Here's how the part is built. I have some questions about the finished solid (model axes, mm). Face numbers are marked on the shaded views. A direction names the side the tool comes from. Round coordinates to 2 decimals unless told otherwise and drop trailing zeros. Write each loop counter-clockwise with the first axis right and the second up, starting at its lowest first coordinate (ties: lowest second). Pieces come first, ordered by that corner, then holes. Notation, with made-up numbers: (-33, -39.5) -> (-19, -39.5) arc R18 ccw to (-19, -17.5) -> close; hole circle Ø6 at (46.25, 64.5). An arc over 180 degrees is marked (long way). Answer in a Markdown table with one row per item.
from build123d import *

# Parameters (mm, degrees)
SKETCH1_R                               = 5
BOSS_EXTRUDE1_DEPTH                     = 60
BOSS_EXTRUDE2_START                     = 15
BOSS_EXTRUDE2_DEPTH                     = 15
CBORE_FOR_M5_HEX_HEAD_BOLT1_D           = 10
CBORE_FOR_M5_HEX_HEAD_BOLT1_CBORE_D     = 15
CBORE_FOR_M5_HEX_HEAD_BOLT1_CBORE_DEPTH = 8
CHAMFER1_SIZE                           = 20
CUT_EXTRUDE3_DEPTH                      = 338.769583605


with BuildPart() as part:
    # Sketch1 → Boss-Extrude1 (new body)
    with BuildSketch(Plane(origin=(0, 0, 0), x_dir=(1, 0, 0), z_dir=(0, 1, 0))):
        with BuildLine():
            ThreePointArc((0, 15), (-15, 0), (0, -15))
            Line((0, -15), (179, -15))
            Line((179, -15), (191.125444005, -15))
            ThreePointArc((191.125444005, -15), (204.178063227, -15.855513863), (217.007348515, -18.407417371))
            Line((217.007348515, -18.407417371), (260.271455877, -30))
            Line((260.271455877, -30), (285.271455877, -30))
            Line((285.271455877, -30), (285.271455877, -20))
            Line((285.271455877, -20), (255.271455877, -20))
            ThreePointArc((255.271455877, -20), (244.66485416, -15.606601718), (240.271455877, -5))
            Line((240.271455877, -5), (240.271455877, 5))
            ThreePointArc((240.271455877, 5), (244.66485416, 15.606601718), (255.271455877, 20))
            Line((255.271455877, 20), (285.271455877, 20))
            Line((285.271455877, 20), (285.271455877, 30))
            Line((285.271455877, 30), (260.271455877, 30))
            Line((260.271455877, 30), (217.007348515, 18.407417371))
            ThreePointArc((217.007348515, 18.407417371), (204.178063227, 15.855513863), (191.125444005, 15))
            Line((191.125444005, 15), (0, 15))
        make_face()
        with Locations(Location((0, 0, 0), (0, 0, 270))):
            Circle(SKETCH1_R, mode=Mode.SUBTRACT)
    extrude(amount=-BOSS_EXTRUDE1_DEPTH)

    # Sketch4 → Boss-Extrude2 (add)
    with BuildSketch(Plane(origin=(0, -60, 0), x_dir=(1, 0, 0), z_dir=(0, 1, 0)).offset(BOSS_EXTRUDE2_START)):
        with BuildLine():
            Line((260.271455877, -20), (260.271455877, 20))
            Line((260.271455877, 20), (255.271455877, 20))
            ThreePointArc((255.271455877, 20), (244.66485416, 15.606601718), (240.271455877, 5))
            Line((240.271455877, 5), (240.271455877, -5))
            ThreePointArc((240.271455877, -5), (244.66485416, -15.606601718), (255.271455877, -20))
            Line((255.271455877, -20), (260.271455877, -20))
        make_face()
        with BuildLine():
            Line((325.271455877, -18.46), (325.271455877, 18.46))
            ThreePointArc((325.271455877, 18.46), (315.266904712, 35.783134895), (295.262355618, 35.77525085))
            Line((295.262355618, 35.77525085), (285.271455877, 30))
            Line((285.271455877, 30), (285.271455877, 20))
            Line((285.271455877, 20), (260.271455877, 20))
            Line((260.271455877, 20), (260.271455877, -20))
            Line((260.271455877, -20), (285.271455877, -20))
            Line((285.271455877, -20), (285.271455877, -30))
            Line((285.271455877, -30), (295.262355618, -35.77525085))
            ThreePointArc((295.262355618, -35.77525085), (315.266904712, -35.783134895), (325.271455877, -18.46))
        make_face()
    extrude(amount=-BOSS_EXTRUDE2_DEPTH)

    # CBORE for M5 Hex Head Bolt1 (through all)
    with Locations(Plane(origin=(0, -45, 0), x_dir=(1, 0, 0), z_dir=(0, 1, 0))):
        with Locations((265.271455877, 0), (305.271455877, 18.46), (305.271455877, -18.46)):
            CounterBoreHole(CBORE_FOR_M5_HEX_HEAD_BOLT1_D / 2, CBORE_FOR_M5_HEX_HEAD_BOLT1_CBORE_D / 2, CBORE_FOR_M5_HEX_HEAD_BOLT1_CBORE_DEPTH)

    # Chamfer1
    chamfer1_edges = [part.edges().sort_by_distance(p)[0] for p in [
        (285.271455877, 0, -25),
        (285.271455877, 0, 25),
    ]]
    chamfer(chamfer1_edges, length=CHAMFER1_SIZE)

    # Sketch9 → Cut-Extrude3 (cut, through all)
    with BuildSketch(Plane.XY.offset(30)):
        Polygon((-15, 0), (230.271455877, 0), (230.271455877, -26.768114978), (50.271455877, -26.768114978), (50.271455877, -41.766455786), (-14.728544123, -41.766455786), align=None)
        with BuildLine():
            ThreePointArc((141.259972199, -56.766455786), (185.683449524, -56.91600014), (230, -60))
            Line((230, -60), (-15, -60))
            Line((-15, -60), (-14.728544123, -56.766455786))
            Line((-14.728544123, -56.766455786), (141.259972199, -56.766455786))
        make_face()
    extrude(amount=-CUT_EXTRUDE3_DEPTH, mode=Mode.SUBTRACT)


solid = part.part
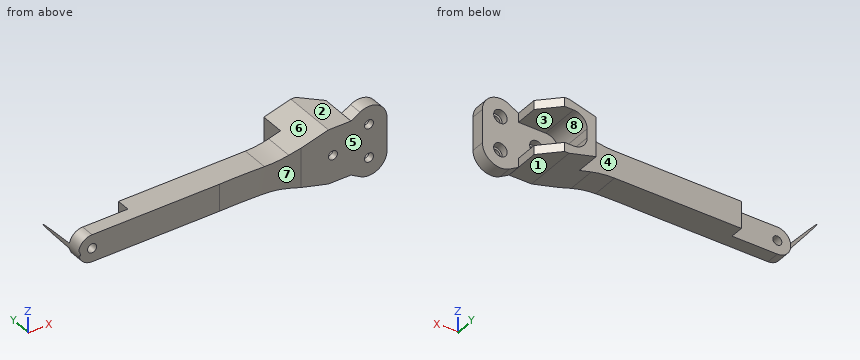
1) I want a section at D-D, the plane x = 57. List the corners of the cut face in (y, z) for me.
Response:
| item | result |
|---|---|
| outline | (-56.77, -15) -> (-26.77, -15) -> (-26.77, 15) -> (-56.77, 15) -> close |
2) I want a section at B-B, the plane y = -16. List the corners of the cut face in (x, z) for me.
Response:
| item | result |
|---|---|
| outline | (-14.9, -1.76) -> (-14.9, 1.76) arc R15 ccw to start; (230.27, -21.96) -> (260.27, -30) -> (281.27, -30) -> (281.27, -20) -> (255.27, -20) arc R15 cw to (240.27, -5) -> (240.27, 5) arc R15 cw to (255.27, 20) -> (281.27, 20) -> (281.27, 30) -> (260.27, 30) -> (230.27, 21.96) -> close |
3) Which directions (+Z, -Z, +X, -X, +Y, -Y) give clear straight access to the entire face, cutting with the end or side of a thin tool? Please do the marked faces 1, 2, 3, 4 and 5.
Response:
| item | result |
|---|---|
| face 1 | -Z, -X, +Y, -Y |
| face 2 | +Z, -X, +Y, -Y |
| face 3 | +X, +Y |
| face 4 | +Z, -Z, +Y |
| face 5 | +Z, -Z, +X, -X, -Y |
4) I need wall thicknesses on line 1 (Z direction, x = 13, y = -44); line 2 (Y direction, x = 9.5, z = -9.5); line 3 (Y direction, x = 68.5, z = -10). Which ranges of each line are inside material? Lowest first, please. Write a range as [from, to].
Response:
| item | result |
|---|---|
| line 1 | z = [-15, 15] |
| line 2 | y = [-56.77, -41.77] |
| line 3 | y = [-56.77, -26.77] |
5) We'd pull the mould along X, two halves only. Please class the marked faces 6, 7 and 8: +X half, -X half, draft (parallel to the pull), parting line (faces both ways), or undercut.
Response:
| item | result |
|---|---|
| face 6 | -X half |
| face 7 | undercut |
| face 8 | +X half |
6) For pin 1 (2 mm diameter, centred on x = 123, y = -34.5, fed in from -Z); pin 2 (24 mm diameter, centred on x = 267, y = -29.5, fed in from +Z); pin 3 (12 mm diameter, centred on y = -31.5, z = -20, fed in from -X); pin 4 (9 mm diameter, centred on x = 305.27, z = -18.46, fed in from -Y), each with a flat end and sliding along its axis, tell me the tip position at first contact or that it passes through.
Response:
| item | result |
|---|---|
| pin 1 | stops at z = -15 |
| pin 2 | stops at z = 30 |
| pin 3 | stops at x = 50.27 |
| pin 4 | passes through |
7) I want a section at C-C, the plane x = 281. List the corners of the cut face in (y, z) for me, and give its area (3 significant figures).
Response:
| item | result |
|---|---|
| outline | (-60, -30) -> (-15.73, -30) -> (-15.73, -20) -> (-45, -20) -> (-45, 20) -> (-15.73, 20) -> (-15.73, 30) -> (-60, 30) -> close |
| area | 1,490 mm^2 |
8) I want a section at A-A, the plane z = 0. List the corners of the cut face in (x, y) for me, and give its area (3 significant figures).
Response:
| item | result |
|---|---|
| outline | (-15, -60) -> (-14.73, -56.77) -> (-5, -56.77) -> (-5, -41.77) -> (-14.73, -41.77) -> (-15, 0) -> close; (5, -56.77) -> (141.26, -56.77) arc R672.07 cw to (230, -60) -> (260.27, -60) -> (260.27, -53) -> (257.77, -53) -> (257.77, -45) -> (240.27, -45) -> (240.27, 0) -> (230.27, 0) -> (230.27, -26.77) -> (50.27, -26.77) -> (50.27, -41.77) -> (5, -41.77) -> close; (270.27, -60) -> (325.27, -60) -> (325.27, -45) -> (272.77, -45) -> (272.77, -53) -> (270.27, -53) -> close |
| area | 7,980 mm^2 |
